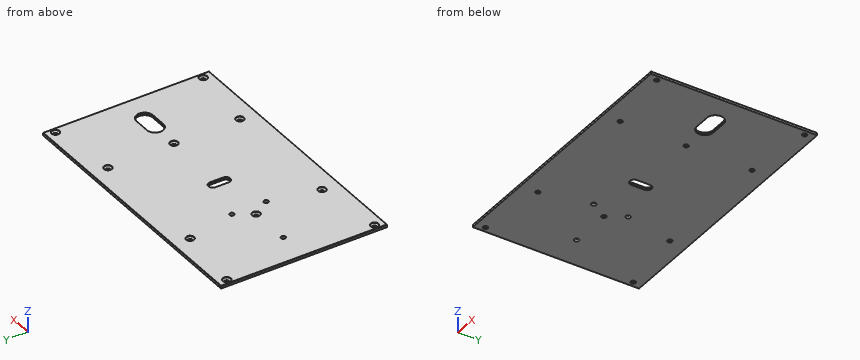
```python
from build123d import *

# Parameters (mm, degrees)
SKETCH1_W                                      = 206
SKETCH1_H                                      = 126
SKETCH1_R                                      = 1.75
BOSS_EXTRUDE1_DEPTH                            = 2
CUT_EXTRUDE1_REACH                             = 217.55
SKETCH2_R                                      = 1.75
CUT_EXTRUDE2_REACH                             = 217.55
CSK_FOR_M3_FLAT_HEAD_MACHINE_SCREW1_AT_2_COUNT = 2
CSK_FOR_M3_FLAT_HEAD_MACHINE_SCREW1_AT_2_PITCH = 51.848336521
CSK_FOR_M3_FLAT_HEAD_MACHINE_SCREW1_AT_3_COUNT = 2
CSK_FOR_M3_FLAT_HEAD_MACHINE_SCREW1_AT_3_PITCH = 76.08054942
CSK_FOR_M3_FLAT_HEAD_MACHINE_SCREW1_AT_4_COUNT = 2
CSK_FOR_M3_FLAT_HEAD_MACHINE_SCREW1_AT_4_PITCH = 117.848419591
CSK_FOR_M3_FLAT_HEAD_MACHINE_SCREW1_AT_5_COUNT = 2
CSK_FOR_M3_FLAT_HEAD_MACHINE_SCREW1_AT_5_PITCH = 112
CSK_FOR_M3_FLAT_HEAD_MACHINE_SCREW1_AT_6_COUNT = 2
CSK_FOR_M3_FLAT_HEAD_MACHINE_SCREW1_AT_6_PITCH = 146.622815414
CSK_FOR_M3_FLAT_HEAD_MACHINE_SCREW1_AT_7_COUNT = 2
CSK_FOR_M3_FLAT_HEAD_MACHINE_SCREW1_AT_7_PITCH = 198
CSK_FOR_M3_FLAT_HEAD_MACHINE_SCREW1_AT_8_COUNT = 2
CSK_FOR_M3_FLAT_HEAD_MACHINE_SCREW1_AT_8_PITCH = 227.481867409
CSK_FOR_M3_FLAT_HEAD_MACHINE_SCREW1_AT_9_COUNT = 2
CSK_FOR_M3_FLAT_HEAD_MACHINE_SCREW1_AT_9_PITCH = 156.838292518
CSK_FOR_M3_FLAT_HEAD_MACHINE_SCREW1_AT_1_COUNT = 2
CSK_FOR_M3_FLAT_HEAD_MACHINE_SCREW1_AT_1_PITCH = 180.826574374
CHAMFER1_SIZE                                  = 0.25


with BuildPart() as part:
    # Sketch1 → Boss-Extrude1 (new body)
    with BuildSketch(Plane.XY):
        with Locations((74, -60)):
            Rectangle(SKETCH1_W, SKETCH1_H)
        with Locations((-25, -4)):
            Circle(SKETCH1_R, mode=Mode.SUBTRACT)
        with Locations((26.5, -10)):
            Circle(SKETCH1_R, mode=Mode.SUBTRACT)
        with Locations((121.5, -10)):
            Circle(SKETCH1_R, mode=Mode.SUBTRACT)
        with Locations((173, -4)):
            Circle(SKETCH1_R, mode=Mode.SUBTRACT)
        with Locations((173, -116)):
            Circle(SKETCH1_R, mode=Mode.SUBTRACT)
        with Locations((121.5, -60)):
            Circle(SKETCH1_R, mode=Mode.SUBTRACT)
        with Locations((121.5, -110)):
            Circle(SKETCH1_R, mode=Mode.SUBTRACT)
        with Locations((26.5, -110)):
            Circle(SKETCH1_R, mode=Mode.SUBTRACT)
        with Locations((26.5, -60)):
            Circle(SKETCH1_R, mode=Mode.SUBTRACT)
        with Locations((-25, -116)):
            Circle(SKETCH1_R, mode=Mode.SUBTRACT)
    extrude(amount=BOSS_EXTRUDE1_DEPTH)

    # Sketch2 → Cut-Extrude1 (cut, up to next)
    with BuildSketch(Plane.XY.offset(2), mode=Mode.PRIVATE) as cut_extrude1_sk1:
        with Locations((34.621837413, -47)):
            Circle(SKETCH2_R)
    cut_extrude1_tool1 = extrude(cut_extrude1_sk1.sketch, amount=-CUT_EXTRUDE1_REACH, mode=Mode.PRIVATE) & part.part
    # Sketch2 → Cut-Extrude1 (cut, up to next)
    with BuildSketch(Plane.XY.offset(2), mode=Mode.PRIVATE) as cut_extrude1_sk2:
        with Locations((34.621837413, -73)):
            Circle(SKETCH2_R)
    cut_extrude1_tool2 = extrude(cut_extrude1_sk2.sketch, amount=-CUT_EXTRUDE1_REACH, mode=Mode.PRIVATE) & part.part
    # Sketch2 → Cut-Extrude1 (cut, up to next)
    with BuildSketch(Plane.XY.offset(2), mode=Mode.PRIVATE) as cut_extrude1_sk3:
        with Locations((-5, -60)):
            Circle(SKETCH2_R)
    cut_extrude1_tool3 = extrude(cut_extrude1_sk3.sketch, amount=-CUT_EXTRUDE1_REACH, mode=Mode.PRIVATE) & part.part
    add(cut_extrude1_tool1.solids().sort_by_distance((34.621837, -47, 2))[0], mode=Mode.SUBTRACT)
    add(cut_extrude1_tool2.solids().sort_by_distance((34.621837, -73, 2))[0], mode=Mode.SUBTRACT)
    add(cut_extrude1_tool3.solids().sort_by_distance((-5, -60, 2))[0], mode=Mode.SUBTRACT)

    # Sketch7 → Cut-Extrude2 (cut, up to next)
    with BuildSketch(Plane.XY.offset(2), mode=Mode.PRIVATE) as cut_extrude2_sk1:
        with BuildLine():
            Line((72, -55), (72, -65))
            ThreePointArc((72, -65), (69, -68), (66, -65))
            Line((66, -65), (66, -55))
            ThreePointArc((66, -55), (69, -52), (72, -55))
        make_face()
    cut_extrude2_tool1 = extrude(cut_extrude2_sk1.sketch, amount=-CUT_EXTRUDE2_REACH, mode=Mode.PRIVATE) & part.part
    # Sketch7 → Cut-Extrude2 (cut, up to next)
    with BuildSketch(Plane.XY.offset(2), mode=Mode.PRIVATE) as cut_extrude2_sk2:
        with BuildLine():
            Line((143.25, -54), (155.25, -54))
            ThreePointArc((155.25, -54), (161.25, -60), (155.25, -66))
            Line((155.25, -66), (143.25, -66))
            ThreePointArc((143.25, -66), (137.25, -60), (143.25, -54))
        make_face()
    cut_extrude2_tool2 = extrude(cut_extrude2_sk2.sketch, amount=-CUT_EXTRUDE2_REACH, mode=Mode.PRIVATE) & part.part
    add(cut_extrude2_tool1.solids().sort_by_distance((69, -60, 2))[0], mode=Mode.SUBTRACT)
    add(cut_extrude2_tool2.solids().sort_by_distance((149.25, -60, 2))[0], mode=Mode.SUBTRACT)

    # Sketch4 → CSK for M3 Flat Head Machine Screw1 (revolve, cut)
    with BuildSketch(Plane(origin=(-25, -4, 2), x_dir=(0, -1, 0), z_dir=(1, 0, 0))):
        Polygon((0, 0), (0, 2), (1.75, 2), (1.75, 1.65), (3, 0.4), (3, 0), align=None)
    csk_for_m3_flat_head_machine_screw1 = revolve(axis=Axis((-25, -4, 8.35), (0, 0, -1)), mode=Mode.SUBTRACT)

    # CSK for M3 Flat Head Machine Screw1 at 2: CSK for M3 Flat Head Machine Screw1 ×2
    with Locations(*[Vector(0.9932816259031161, -0.11572213117317788, 0) * (i * CSK_FOR_M3_FLAT_HEAD_MACHINE_SCREW1_AT_2_PITCH) for i in range(1, CSK_FOR_M3_FLAT_HEAD_MACHINE_SCREW1_AT_2_COUNT)]):
        add(csk_for_m3_flat_head_machine_screw1, mode=Mode.SUBTRACT)

    # CSK for M3 Flat Head Machine Screw1 at 3: CSK for M3 Flat Head Machine Screw1 ×2
    with Locations(*[Vector(0.6769141441909728, -0.7360619820329011, 0) * (i * CSK_FOR_M3_FLAT_HEAD_MACHINE_SCREW1_AT_3_PITCH) for i in range(1, CSK_FOR_M3_FLAT_HEAD_MACHINE_SCREW1_AT_3_COUNT)]):
        add(csk_for_m3_flat_head_machine_screw1, mode=Mode.SUBTRACT)

    # CSK for M3 Flat Head Machine Screw1 at 4: CSK for M3 Flat Head Machine Screw1 ×2
    with Locations(*[Vector(0.4370020419358412, -0.8994605134990115, 0) * (i * CSK_FOR_M3_FLAT_HEAD_MACHINE_SCREW1_AT_4_PITCH) for i in range(1, CSK_FOR_M3_FLAT_HEAD_MACHINE_SCREW1_AT_4_COUNT)]):
        add(csk_for_m3_flat_head_machine_screw1, mode=Mode.SUBTRACT)

    # CSK for M3 Flat Head Machine Screw1 at 5: CSK for M3 Flat Head Machine Screw1 ×2
    with Locations(*[(0, -i * CSK_FOR_M3_FLAT_HEAD_MACHINE_SCREW1_AT_5_PITCH, 0) for i in range(1, CSK_FOR_M3_FLAT_HEAD_MACHINE_SCREW1_AT_5_COUNT)]):
        add(csk_for_m3_flat_head_machine_screw1, mode=Mode.SUBTRACT)

    # CSK for M3 Flat Head Machine Screw1 at 6: CSK for M3 Flat Head Machine Screw1 ×2
    with Locations(*[Vector(0.9991623717366304, -0.04092132580491247, 0) * (i * CSK_FOR_M3_FLAT_HEAD_MACHINE_SCREW1_AT_6_PITCH) for i in range(1, CSK_FOR_M3_FLAT_HEAD_MACHINE_SCREW1_AT_6_COUNT)]):
        add(csk_for_m3_flat_head_machine_screw1, mode=Mode.SUBTRACT)

    # CSK for M3 Flat Head Machine Screw1 at 7: CSK for M3 Flat Head Machine Screw1 ×2
    with Locations(*[(i * CSK_FOR_M3_FLAT_HEAD_MACHINE_SCREW1_AT_7_PITCH, 0, 0) for i in range(1, CSK_FOR_M3_FLAT_HEAD_MACHINE_SCREW1_AT_7_COUNT)]):
        add(csk_for_m3_flat_head_machine_screw1, mode=Mode.SUBTRACT)

    # CSK for M3 Flat Head Machine Screw1 at 8: CSK for M3 Flat Head Machine Screw1 ×2
    with Locations(*[Vector(0.8703990443501523, -0.4923469341778639, 0) * (i * CSK_FOR_M3_FLAT_HEAD_MACHINE_SCREW1_AT_8_PITCH) for i in range(1, CSK_FOR_M3_FLAT_HEAD_MACHINE_SCREW1_AT_8_COUNT)]):
        add(csk_for_m3_flat_head_machine_screw1, mode=Mode.SUBTRACT)

    # CSK for M3 Flat Head Machine Screw1 at 9: CSK for M3 Flat Head Machine Screw1 ×2
    with Locations(*[Vector(0.934083109729549, -0.3570556596918405, 0) * (i * CSK_FOR_M3_FLAT_HEAD_MACHINE_SCREW1_AT_9_PITCH) for i in range(1, CSK_FOR_M3_FLAT_HEAD_MACHINE_SCREW1_AT_9_COUNT)]):
        add(csk_for_m3_flat_head_machine_screw1, mode=Mode.SUBTRACT)

    # CSK for M3 Flat Head Machine Screw1 at 1: CSK for M3 Flat Head Machine Screw1 ×2
    with Locations(*[Vector(0.8101685302992528, -0.5861970253359775, 0) * (i * CSK_FOR_M3_FLAT_HEAD_MACHINE_SCREW1_AT_1_PITCH) for i in range(1, CSK_FOR_M3_FLAT_HEAD_MACHINE_SCREW1_AT_1_COUNT)]):
        add(csk_for_m3_flat_head_machine_screw1, mode=Mode.SUBTRACT)

    # Chamfer1
    chamfer1_edges = [part.edges().sort_by_distance(p)[0] for p in [
        (177, -60, 2),
        (74, 3, 2),
        (-29, -60, 2),
        (-29, 3, 1),
        (177, 3, 1),
        (177, -123, 1),
        (-29, -123, 1),
        (69, -52, 2),
        (66, -60, 2),
        (69, -68, 2),
        (72, -60, 2),
        (66, -60, 0),
        (69, -52, 0),
        (72, -60, 0),
        (69, -68, 0),
        (137.25, -60, 2),
        (149.25, -66, 2),
        (161.25, -60, 2),
        (149.25, -54, 2),
        (149.25, -66, 0),
        (137.25, -60, 0),
        (149.25, -54, 0),
        (161.25, -60, 0),
        (74, -123, 2),
    ]]
    chamfer(chamfer1_edges, length=CHAMFER1_SIZE)


solid = part.part
```
Check sheet for the modelled part. Datum: model origin and axes. Units: mm. Coordinates: 2 decimals unless noted, no trailing zeros. Write item = value, one per line. Start each with the question number.
1) Cross-section at A-A (z = 1). State how many separate pieces and enclosed holes the cut face has, then the cut area to 3 significant figures.
2) Material ranges on L1, parallel to X at y = -116, z = 0.25; L2, parallel to Y at x = -25, z = 0.2; L3, parallel to X at y = -10, z = 0.3, recorded low to high.
3) Go/stop test with flat-tipped pins: P1, Ø4, axis at x = 26.5, y = -10, coming from the +Z side; P2, Ø5, axis at x = 121.5, y = -60, coming from the +Z side; P3, Ø5.5, axis at x = 121.5, y = -110, coming from the +Z side. Record where each tip stops, or that it passes through.
Ans:
q1.separate_pieces = 1
q1.enclosed_holes = 15
q1.area = 25,400 mm²
q2.L1 = -29 to -26.75, -23.25 to 171.25, 174.75 to 177
q2.L2 = -123 to -117.75, -114.25 to -5.75, -2.25 to 3
q2.L3 = -29 to 24.75, 28.25 to 119.75, 123.25 to 177
q3.P1 = 0.6
q3.P2 = 1.1
q3.P3 = 1.35
